For this review, take the finished solid that the model builds, in its own axes (mm). Face numbers are marked on the shaded views. A direction names the side the tool comes from. Give positions to 0.01 mm unless a question says otherwise; leave off trailing zeros. Order: outer loops, then holes, each group sorted by start corner. A loop starts at its lowest first (then second) coordinate and runs counter-clockwise, first axis right, second up.
Autodesk Inventor part; units mm, degrees
ref_plane "Work Plane2" through (0, 0, 2.5) normal (0, 0, 1) x (1, 0, 0)
ref_plane "Work Plane8" through (0, 0, 0) normal (0.9510565, 0.309017, 0) x (0, 0, 1)
ref_plane "Work Plane9" through (0, 0, 0) normal (1, 0, 0) x (0, 1, 0)
sketch "Sketch1" plane through (0, 0, 0) normal (0, 0, 1) x (1, 0, 0)
  circle A0 centre (0, 0) radius 12
  dimension "d0" = 24
extrude "Extrusion1" add sketch "Sketch1" along normal blind 5
ref_plane "Work Plane2" through (0, 0, 2.5) normal (0, 0, 1) x (1, 0, 0)
sketch "Sketch2" plane through (0, 0, 0) normal (0, 0, -1) x (-1, 0, 0)
  circle A0 centre (0, 0) radius 12
  circle A1 centre (0, 0) radius 10
  dimension "d3" = 20
surface extrude "Pitch Diameter" sketch "Sketch2" against normal through all shown no curves A1
ref_plane "Work Plane8" through (0, 0, 0) normal (0.9510565, 0.309017, 0) x (0, 0, 1)
ref_plane "Work Plane9" through (0, 0, 0) normal (1, 0, 0) x (0, 1, 0)
spur gear teeth "Spur Gear" teeth 10 pitch diameter 20 tip diameter 24 root diameter 15 face width 5 start plane through (0, 0, 0) normal (0, 0, -1) x (-1, 0, 0)
equation "\"d0\" = da_da"
equation "\"d1\" = da_b"
equation "\"d3\" = da_d"
properties part number "Spur Gear1" material "Steel"
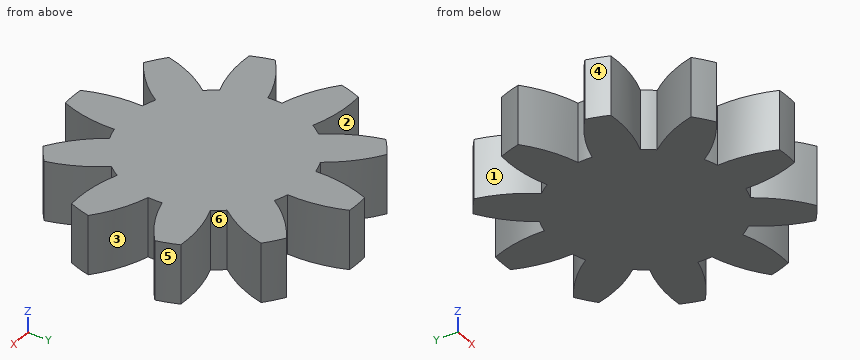
1) Clearance check with a flat-ended pin moving along its axis: pin 1 (3 mm diameter, centred on x = 2, z = 1.5, fed in from -Y). State where the tip first meets the part, or that it passes through.
Answer sheet:
pin 1: stops at y = -11.99
2) To check wall thickness, follow line 1 (Y direction, x = -7, z = 3.6); line 2 (X direction, y = 9.25, z = 3.2); line 3 (Y direction, x = 6, z = 2.8). State the ranges of each line that lie inside material, in increasing order.
Answer sheet:
line 1: y = -9.75 to -6.92, -4.13 to 4.13, 6.92 to 9.75
line 2: x = -7.64 to -4.92, -1.67 to 1.67, 4.92 to 7.64
line 3: y = -10.06 to -5.26, -4.5 to 4.5, 5.26 to 10.06
3) Tool access review of the marked faces 1, 2 and 3: name each direction out of +Z, -Z, +X, -X, +Y, -Y from which nothing blocks a thin tool from reaching the whole face with its end or side.
Answer sheet:
face 1: +Z, -Z, -X
face 2: +Z, -Z
face 3: +Z, -Z, +X
4) We need section C-C on y = -8.75. Give the boundary of the cut face in (x, z).
Answer sheet:
outline: (-7.7, 0) - (-4.37, 0) - (-4.37, 5) - (-7.7, 5) - close; (-1.72, 0) - (1.72, 0) - (1.72, 5) - (-1.72, 5) - close; (4.37, 0) - (7.7, 0) - (7.7, 5) - (4.37, 5) - close
5) We need section D-D on x = 4.75. Give the boundary of the cut face in (y, z).
Answer sheet:
outline: (-9.1, 0) - (9.1, 0) - (9.1, 5) - (-9.1, 5) - close
6) We need section B-B on y = 8. Give the boundary of the cut face in (x, z).
Answer sheet:
outline: (-7.45, 0) - (-3.67, 0) - (-3.67, 5) - (-7.45, 5) - close; (-1.76, 0) - (1.76, 0) - (1.76, 5) - (-1.76, 5) - close; (3.67, 0) - (7.45, 0) - (7.45, 5) - (3.67, 5) - close
7) Draft analysis for pull direction Y (two halves, no side actions). For the marked faces 4, 5 and 6, state which applies: +Y half, -Y half, draft (parallel to the pull), parting line (faces both ways), or undercut.
Answer sheet:
face 4: -Y half
face 5: +Y half
face 6: undercut
8) We need section A-A on x = -10.5. Give the boundary of the cut face in (y, z), then the cut area to 3 significant figures.
Answer sheet:
outline: (-4.62, 0) - (-1.94, 0) - (-1.94, 5) - (-4.62, 5) - close; (1.94, 0) - (4.62, 0) - (4.62, 5) - (1.94, 5) - close
area: 26.8 mm2
